Autodesk Inventor part; units mm, degrees
ref_plane "YZ Plane" through (0, 0, 0) normal (1, 0, 0) x (0, 1, 0)
ref_plane "XZ Plane" through (0, 0, 0) normal (0, 1, 0) x (-1, 0, 0)
ref_plane "XY Plane" through (0, 0, 0) normal (0, 0, 1) x (1, 0, 0)
sketch "Sketch1" plane through (0, 0, 0) normal (0, 0, 1) x (1, 0, 0)
  circle A0 centre (0, 0) radius 40
  circle A1 centre (0, 0) radius 50
  dimension "d0" = 80
  dimension "d1" = 100
extrude "Extrusion1" add sketch "Sketch1" along normal blind 50
sketch "Sketch2" plane through (0, 0, 0) normal (0, 0, -1) x (-1, 0, 0)
  circle A0 centre (0, 0) radius 45.1
  circle A1 centre (0, 0) radius 50
  dimension "d5" = 90.2
extrude "Extrusion2" add sketch "Sketch2" along normal blind 10
sketch "Sketch3" plane through (0, 0, 0) normal (0, 1, 0) x (-1, 0, 0)
  line L0 (-50, -10) -> (50, -10) construction
  point P0 (0, 0)
  point P1 (0, -5)
  dimension "d8" = 5
hole "Hole1" at (0, 0, -5) direction (0, 1, 0) diameter 3.4 end through all
pattern_circular "Circular Pattern1" count 3 over 360 about axis through (0, 0, -10) along (0, 0, 1) of "Hole1"
fillet "Fillet1" radius 5 2 edges at (-50, 0, 50) (-40, 0, 50)
sketch "Sketch4" plane through (0, 0, 0) normal (0, 1, 0) x (-1, 0, 0)
  point P0 (0, 0)
  point P1 (0, 40)
  point P2 (0, 10)
  dimension "d19" = 10
  dimension "d20" = 40
hole "Hole2" at (0, 0, 40) at (0, 0, 10) direction (0, -1, 0) diameter 2.459 end through all
properties part number "Nose"
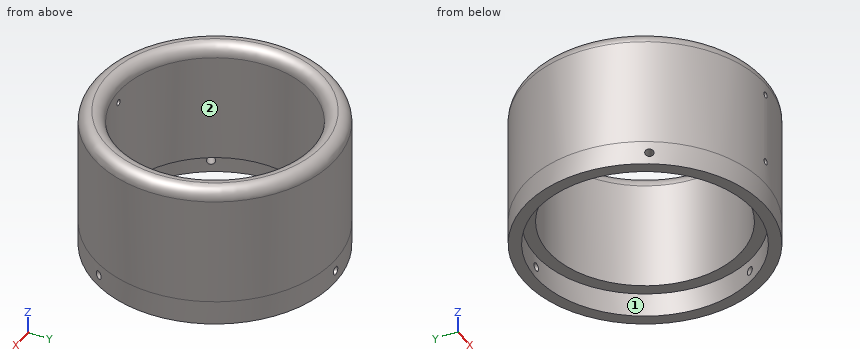
Design review of the part built by this model. Coordinates are the model's own, in mm. Face numbers are marked on the shaded views. A direction names the side the tool comes from. Coordinates: 2 decimals unless noted, no trailing zeros. Order: outer loops, then holes, each group sorted by start corner. A loop starts at its lowest first (then second) coordinate and runs counter-clockwise, first axis right, second up. Notation, with made-up numbers: M 50,-3.75 L 55,-3.75 A21 cw 55,2.25 Z; hole C -8.5,-30 d7. An arc over 180 degrees is marked long. Answer as a JSON object with one key per item and string values. Group by question number.
1) Add section C-C, the plane z = -5. Write out the cut boundary in (x, y).
2) Wall thickness on L1, parallel to Z at x = 0, y = -45; L2, parallel to Z at x = 0, y = -45.5; L3, parallel to Y at x = 0, z = -2: over which ranges is each line inside the solid? List them lowest first.
3) Add section A-A, the plane x = 0. Count the separate pieces of the cut face and the enclosed holes in it, then the cut area to 3 significant figures.
4) Tool access review of the marked faces 1 and 2: name each direction out of +Z, -Z, +X, -X, +Y, -Y from which nothing blocks a thin tool from reaching the whole face with its end or side.
5) For pin 1 (1.5 mm diameter, centred on y = 28, z = 36.5, fed in from +X); pin 2 (8 mm diameter, centred on y = -25, z = 32, fed in from -X); pin 3 (6 mm diameter, centred on x = 39, z = 7, fed in from +Y), all flat-tipped, find the tip position at first contact; note any pin that passes through.
6) Add section D-D, the plane z = 18.5. Write out the cut boundary in (x, y), then the cut area to 3 significant figures.
Computed values:
{
 "1": {"outline": "M -44.13,-23.51 L -39.88,-21.06 A45.1 cw -1.7,45.07 L -1.7,49.97 A50 ccw Z; M -42.43,-26.46 A50 ccw 42.43,-26.46 L 38.18,-24.01 A45.1 cw -38.18,-24.01 Z; M 1.7,45.07 A45.1 cw 39.88,-21.06 L 44.13,-23.51 A50 ccw 1.7,49.97 Z"},
 "2": {"L1": "z = 0 to 8.77, 11.23 to 38.77, 41.23 to 50", "L2": "z = -10 to 8.77, 11.23 to 38.77, 41.23 to 49.97", "L3": "y = -50 to -45.1, 45.1 to 50"},
 "3": {"separate pieces": "5", "enclosed holes": "0", "area": "1,010 mm^2"},
 "4": {"face 1": "-Z", "face 2": "+Z, -Z"},
 "5": {"pin 1": "stops at x = 41.92", "pin 2": "stops at x = -45.38", "pin 3": "stops at y = 34.7"},
 "6": {"outline": "C 0,0 d100; hole C 0,0 d80", "area": "2,830 mm^2"}
}
